from build123d import *

# Parameters (mm, degrees)
EXTRUDE_THIN4_DEPTH = 20
SKETCH2_R           = 5
CUT_EXTRUDE1_DEPTH  = 235


# Read off the part's stored shape, not the designer's step: Extrude-Thin4
with BuildPart() as part:
    # Extrude-Thin4 outline → Extrude-Thin4 (new body)
    with BuildSketch(Plane.XY):
        Polygon((201.180339887, 5), (1.180339887, 105), (-25, 105), (-25, 95), (-1.180339887, 95), (188.819660113, 0), (-1.180339887, -95), (-25, -95), (-25, -105), (1.180339887, -105), (201.180339887, -5), (225, -5), (225, 5), align=None)
    extrude(amount=EXTRUDE_THIN4_DEPTH)

    # Sketch2 → Cut-Extrude1 (cut)
    with BuildSketch(Plane.XZ.offset(105)):
        with Locations(Location((-11.319660113, 10, 0), (0, 0, 270))):
            Circle(SKETCH2_R)
        with Locations(Location((213.680339887, 10, 0), (0, 0, 180))):
            Circle(SKETCH2_R)
    extrude(amount=-CUT_EXTRUDE1_DEPTH, mode=Mode.SUBTRACT)


solid = part.part
The listing builds one solid part. Answer for the finished solid, in the listing's coordinates (mm). A direction names the side the tool comes from. Round coordinates to 2 decimals unless told otherwise and drop trailing zeros. Write each loop counter-clockwise with the first axis right and the second up, starting at its lowest first coordinate (ties: lowest second). Pieces come first, ordered by that corner, then holes. Notation, with made-up numbers: M 14,45 L 39,45 A23 ccw 39,57 Z; hole C 82.25,4.25 d1. An arc over 180 degrees is marked long. Write each question's results on one line, items separated by ' | '. Start each with the question number.
Item 1: Straight lines are drawn through the part: L1, parallel to Y at x = -14, z = 1.25; L2, parallel to X at y = 98, z = 10; L3, parallel to Y at x = 50.5, z = 14. For each, find the intervals that lie inside material, in ascending order. Write a range as [from, to].
Item 2: For a pull along X with two mould halves and no side action, classify faces 1 (the face through (-15.9, 95, 7.6)), 2 (the face through (99.78, -55.7, 9.86)), 3 (the face through (95.15, -46.835, 9.86)), 4 (the face through (217.65, -0.07, 13.04)) as pulls with the +X half, pulls with the -X half, needs draft (parallel to the pull), parting line crosses it, or undercut.
Item 3: Flat-ended cylindrical pins translate along their axes: pin 1 Ø5 at (x, z) = (145, 6) entering from +Y; pin 2 Ø12 at (x, y) = (104, -34.5) entering from +Z; pin 3 Ø8 at (x, z) = (163.5, 2.5) entering from +Y; pin 4 Ø1 at (y, z) = (71.5, 15.5) entering from -X. Find the tip coordinate at first contact, or state that the pin passes through.
Item 4: For faces 5 (the face through (211, 5, 5)), 6 (the face through (210, -5, 5)), 7 (the face through (-18, -95, 10)), determine the directions among +Z, -Z, +X, -X, +Y, -Y from which every point of the face is accessible in a straight line to the end or side of a thin tool.
Item 5: A cutting plane is placed at A-A on z = 10. Write down the section's boundary in (x, y), and give its area (3 significant figures).
Item 6: A cutting plane is placed at D-D on y = 34.5. Write down the section's boundary in (x, z), and give its area (3 significant figures).
Item 7: A cutting plane is placed at B-B on x = 40.5. Write down the section's boundary in (y, z).
Item 8: A cutting plane is placed at C-C on x = 197.5. Write down the section's boundary in (y, z), and give its area (3 significant figures).
Check sheet entries:
1) L1: [-105, -95], [95, 105] | L2: [-25, -16.32], [-6.32, 15.18] | L3: [-80.34, -69.16], [69.16, 80.34]
2) face 1: needs draft | face 2: pulls with the +X half | face 3: pulls with the -X half | face 4: undercut
3) pin 1: y = 34.34 | pin 2: through | pin 3: y = 25.84 | pin 4: x = 44.82
4) face 5: +Z, -Z, +X, +Y | face 6: +Z, -Z, +X, -Y | face 7: +Z, -Z, -X
5) outline: M -25,-105 L -16.32,-105 L -16.32,-95 L -25,-95 Z; M -25,95 L -16.32,95 L -16.32,105 L -25,105 Z; M -6.32,-105 L 1.18,-105 L 201.18,-5 L 208.68,-5 L 208.68,5 L 201.18,5 L 1.18,105 L -6.32,105 L -6.32,95 L -1.18,95 L 188.82,0 L -1.18,-95 L -6.32,-95 Z; M 218.68,-5 L 225,-5 L 225,5 L 218.68,5 Z | area: 4,860 mm²
6) outline: M 119.82,0 L 142.18,0 L 142.18,20 L 119.82,20 Z | area: 447 mm²
7) outline: M -85.34,0 L -74.16,0 L -74.16,20 L -85.34,20 Z; M 74.16,0 L 85.34,0 L 85.34,20 L 74.16,20 Z
8) outline: M -6.84,0 L 6.84,0 L 6.84,20 L -6.84,20 Z | area: 274 mm²
